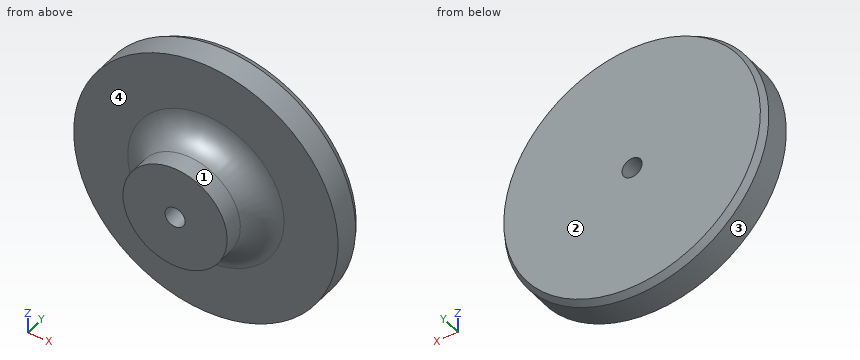
```python
from build123d import *

# Parameters (mm, degrees)
CHAMFER1_SIZE  = 0.381
CHAMFER1_SIZE2 = 0.659911358


with BuildPart() as part:
    # Sketch1 → Revolve1 (revolve)
    with BuildSketch(Plane(origin=(0, 0, 0), x_dir=(0, 0, -1), z_dir=(1, 0, 0))):
        with BuildLine():
            Line((-0.9779, 0), (-0.9779, 7.62))
            Line((-0.9779, 7.62), (-12.8905, 7.62))
            Line((-12.8905, 7.62), (-12.8905, 4.445))
            Line((-12.8905, 4.445), (-7.62, 4.445))
            ThreePointArc((-7.62, 4.445), (-5.823948776, 3.701051224), (-5.08, 1.905))
            Line((-5.08, 1.905), (-5.08, 0))
            Line((-5.08, 0), (-0.9779, 0))
        make_face()
    revolve(axis=Axis((0, 0, 0), (0, 1, 0)))

    # Chamfer1
    chamfer1_edges = [part.edges().sort_by_distance(p)[0] for p in [
        (0, 7.62, -12.8905),
    ]]
    chamfer1_side = [part.faces().sort_by_distance(p)[0] for p in [
        (0, 7.62, -1.342498399),
    ]]
    chamfer(chamfer1_edges, length=CHAMFER1_SIZE, length2=CHAMFER1_SIZE2, reference=chamfer1_side[0])


solid = part.part
```
Read the model definition and answer for the solid it produces. Units are mm, in the model's axes. Face numbers are marked on the shaded views. A direction names the side the tool comes from. Coordinates: 2 decimals unless noted, no trailing zeros. Order: outer loops, then holes, each group sorted by start corner. A loop starts at its lowest first (then second) coordinate and runs counter-clockwise, first axis right, second up. Notation, with made-up numbers: (89.25, -19.75) - (122.25, -19.75) arc R25 cw to (122.25, -2.75) - close; hole circle Ø1 at (-6, 52.25). An arc over 180 degrees is marked (long way). Answer as a JSON object with one key per item and string values. Group by question number.
Item 1: Flat-ended cylindrical pins translate along their axes: P1, Ø5, axis at x = 4, z = -5, coming from the -Y side; P2, Ø1, axis at x = -4.5, y = 2.5, coming from the -Z side; P3, Ø4, axis at x = -6.5, y = 4.5, coming from the +Z side; P4, Ø3, axis at y = 5.5, z = -2.5, coming from the -X side. Find the tip coordinate at first contact, or state that the pin passes through.
Item 2: Section A-A (z = 0) is taken. Give the vertices of the cut face in (x, y) (1 decimal), plus the area to 3 significant figures.
Item 3: A tool of negligible diameter and unlimited length cuts with its end or side. For the marked faces 3 and 4, from which of +Z, -Z, +X, -X, +Y, -Y can it reach the whole face along a straight path? Write none if from no direction.
Item 4: Section B-B (x = 0) is taken. Give the vertices of the cut face in (y, z) (1 decimal).
Item 5: Consider probe 1 along X at (y, z) = (4.5, 0); probe 2 along Y at (x, z) = (-8.75, -7) (3 decimals); probe 3 along X at (y, z) = (7.25, 3.25). Determine where each line is inside the solid, lowest interval first. Write a range as from..to.
Item 6: The mould has two halves that part along X. Classify the marked faces 1 and 2: +X half, -X half, draft (parallel to the pull), parting line (faces both ways), or undercut.
Item 7: Section C-C (y = 1) is taken. Give the vertices of the cut face in (x, z), plus the area to 3 significant figures.
Results are:
{
 "1": {"P1": "stops at y = 0", "P2": "stops at z = -3.28", "P3": "stops at z = 12.08", "P4": "stops at x = -12.85"},
 "2": {"outline": "(-12.9, 4.4) - (-7.6, 4.4) arc R2.5 cw to (-5.1, 1.9) - (-5.1, 0) - (-1, 0) - (-1, 7.6) - (-12.5, 7.6) - (-12.9, 7) - close; (1, 0) - (5.1, 0) - (5.1, 1.9) arc R2.5 cw to (7.6, 4.4) - (12.9, 4.4) - (12.9, 7) - (12.5, 7.6) - (1, 7.6) - close", "area": "115 mm^2"},
 "3": {"face 3": "+Y, -Y", "face 4": "-Y"},
 "4": {"outline": "(0, -5.1) - (1.9, -5.1) arc R2.5 cw to (4.4, -7.6) - (4.4, -12.9) - (7, -12.9) - (7.6, -12.5) - (7.6, -1) - (0, -1) - close; (0, 1) - (7.6, 1) - (7.6, 12.5) - (7, 12.9) - (4.4, 12.9) - (4.4, 7.6) arc R2.5 cw to (1.9, 5.1) - (0, 5.1) - close"},
 "5": {"probe 1": "x = -12.89..-0.98, 0.98..12.89", "probe 2": "y = 4.445..7.62", "probe 3": "x = -12.3..12.3"},
 "6": {"face 1": "parting line", "face 2": "draft"},
 "7": {"outline": "circle Ø10.16 at (0, 0); hole circle Ø1.96 at (0, 0)", "area": "78.1 mm^2"}
}
